For this review, take the finished solid that the model builds, in its own axes (mm). Give positions to 0.01 mm unless a question says otherwise; leave off trailing zeros. Write each loop counter-clockwise with the first axis right and the second up, starting at its lowest first coordinate (ties: lowest second). Pieces come first, ordered by that corner, then holes. Notation, with made-up numbers: M 19,-11 L 37,-11 A26 cw 37,14 Z; hole C 56,26 d5. An arc over 180 degrees is marked long. Use one line per item in the form item = value. Start each with the question number.
Q1. Clearance check with flat-ended pins moving along their axes: pin 1 Ø4.5 at (x, z) = (-74.84, 78.83) entering from +Y; pin 2 Ø2.5 at (x, z) = (80.1, -78.65) entering from -Y. State where each tip first meets the part, or that it passes through.
Q2. Consider section A-A on x = -51.98. Write out the cut boundary in (y, z), and give its area (3 significant figures).
Q3. Mouldability with a two-part tool opening along X and no side actions: class faces 1 (the cylindrical face through (84, 1, 83)), 2 (the cylindrical face through (81.874, 0.986, 79.753)), 3 (the cylindrical face through (-84, 1, -83)) as released by +X, released by -X, zero draft, split by the parting line, or undercut.
Q4. For probe 1 along X at (y, z) = (0.15, 20.5); probe 2 along Z at (x, y) = (80.1, 0.5); probe 3 along X at (y, z) = (1.8, 21), list the stretches that pass through material, from the lowest coordinate up. Write a range as [from, to].
```python
from build123d import *

# Parameters (mm, degrees)
SKETCH_1_R          = 2
EXTRUDE_1_DEPTH     = 2
SKETCH_3_R          = 2.5
CUT_EXTRUDE_1_DEPTH = 10


with BuildPart() as part:
    # Эскиз1 → Бобышка-Вытянуть1 (new body)
    with BuildSketch(Plane.XZ):
        with BuildLine():
            Line((80, 85), (-80, 85))
            ThreePointArc((-80, 85), (-83.535533906, 83.535533906), (-85, 80))
            Line((-85, 80), (-85, -80))
            ThreePointArc((-85, -80), (-83.535533906, -83.535533906), (-80, -85))
            Line((-80, -85), (80, -85))
            ThreePointArc((80, -85), (83.535533906, -83.535533906), (85, -80))
            Line((85, -80), (85, 80))
            ThreePointArc((85, 80), (83.535533906, 83.535533906), (80, 85))
        make_face()
        with Locations(Location((-74.84, 78.83, 0), (0, 0, 90))):
            Circle(SKETCH_1_R, mode=Mode.SUBTRACT)
        with Locations(Location((80.1, 78.83, 0), (0, 0, 90))):
            Circle(SKETCH_1_R, mode=Mode.SUBTRACT)
        with Locations(Location((80.1, -78.65, 0), (0, 0, 90))):
            Circle(SKETCH_1_R, mode=Mode.SUBTRACT)
        with Locations(Location((-51.98, -78.65, 0), (0, 0, 90))):
            Circle(SKETCH_1_R, mode=Mode.SUBTRACT)
    extrude(amount=-EXTRUDE_1_DEPTH)

    # Эскиз3 → Вырез-Вытянуть1 (cut)
    with BuildSketch(Plane(origin=(0, 2, 0), x_dir=(1, 0, 0), z_dir=(0, 1, 0))):
        with Locations(Location((-27.489542331, -20.533937546, 0), (0, 0, 270))):
            Circle(SKETCH_3_R)
        with Locations(Location((-27.489542331, 70.393970701, 0), (0, 0, 270))):
            Circle(SKETCH_3_R)
        with Locations(Location((27.334465925, -20.533937546, 0), (0, 0, 270))):
            Circle(SKETCH_3_R)
        with Locations(Location((27.334465925, 70.393970701, 0), (0, 0, 270))):
            Circle(SKETCH_3_R)
    extrude(amount=-CUT_EXTRUDE_1_DEPTH, mode=Mode.SUBTRACT)


solid = part.part
```
Working result:
q1.pin_1 = 2
q1.pin_2 = through
q2.outline = M 0,-85 L 2,-85 L 2,-80.65 L 0,-80.65 Z; M 0,-76.65 L 2,-76.65 L 2,85 L 0,85 Z
q2.area = 332 mm²
q3.face_1 = released by +X
q3.face_2 = undercut
q3.face_3 = released by -X
q4.probe_1 = [-85, -29.99], [-24.99, 24.83], [29.83, 85]
q4.probe_2 = [-85, -80.65], [-76.65, 76.83], [80.83, 85]
q4.probe_3 = [-85, -29.95], [-25.03, 24.88], [29.79, 85]
